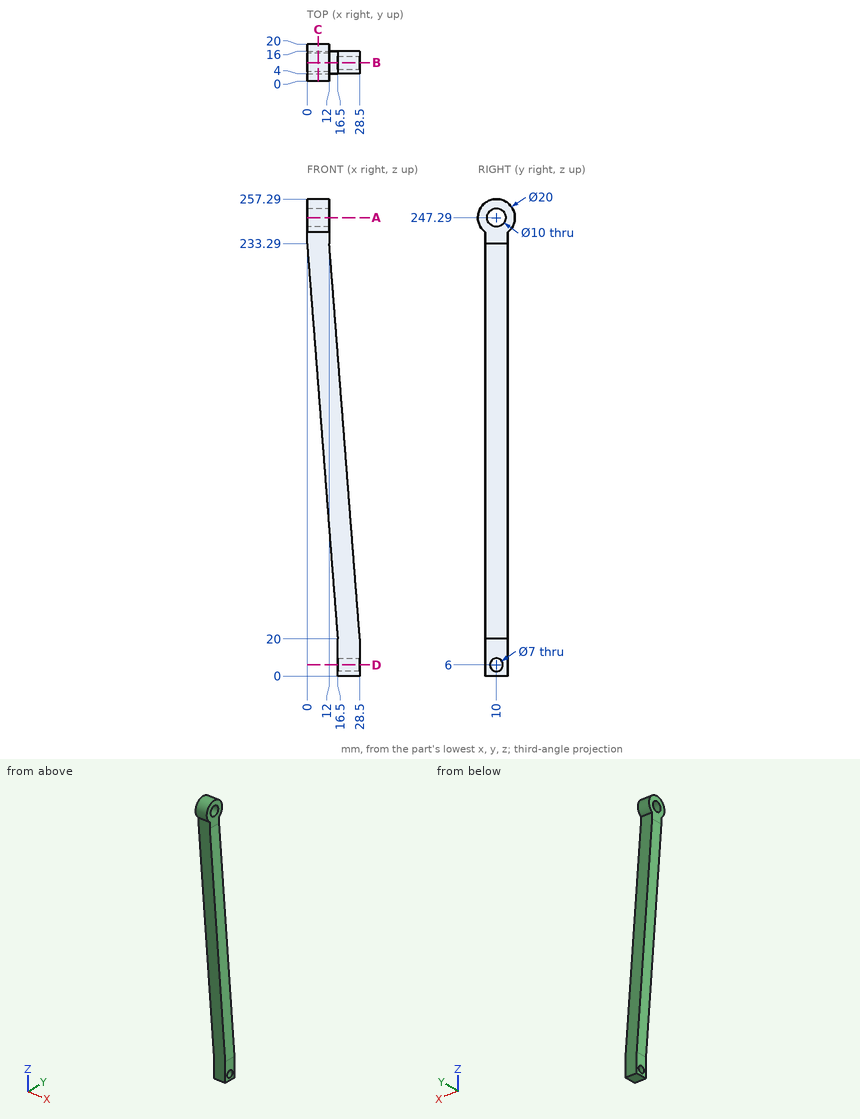
Answer from the drawing. Dimensions are ordinates in mm from the lowest x, y and z of the part. Round coordinates to 2 decimals unless told otherwise and drop trailing zeros. Write each loop counter-clockwise with the first axis right and the second up, starting at its lowest first coordinate (ties: lowest second). Pieces come first, ordered by that corner, then holes.
1. The part is cut by section C-C, the plane x = 6. Determine the outline of the cut face in (y, z).
2. Straight lines are drawn through the part: L1, parallel to Y at x = 25.5, z = 6; L2, parallel to Y at x = 4.5, z = 247.29; L3, parallel to Y at x = 9, z = 141. For each, find the intervals that lie inside material, in ascending order.
3. The part is cut by section D-D, the plane z = 6. Determine the outline of the cut face in (x, y).
4. The part is cut by section A-A, the plane z = 247.29. Determine the outline of the cut face in (x, y), then the cut area to 3 significant figures.
5. The part is cut by section B-B, the plane y = 10. Determine the outline of the cut face in (x, z), then the cut area to 3 significant figures.
6. Given pin 1 Ø3 at (x, z) = (12.5, 163) entering from +Y; pin 2 Ø9.5 at (y, z) = (8, 13.5) entering from -X; pin 3 Ø10 at (y, z) = (10, 246.5) entering from +X, each flat-ended and moving along its own axis, determine where each tip first touches the part or whether it passes through.
Values:
1. outline: (4, 155.73) - (16, 155.73) - (16, 239.29) arc R10 ccw (long way) to (4, 239.29) - close; hole circle Ø10 at (10, 247.29)
2. L1: y = 4 to 6.5, 13.5 to 16
2. L2: y = 0 to 5, 15 to 20
2. L3: y = 4 to 16
3. outline: (16.5, 4) - (28.5, 4) - (28.5, 6.5) - (16.5, 6.5) - close; (16.5, 13.5) - (28.5, 13.5) - (28.5, 16) - (16.5, 16) - close
4. outline: (0, 0) - (12, 0) - (12, 5) - (0, 5) - close; (0, 15) - (12, 15) - (12, 20) - (0, 20) - close
4. area: 120 mm2
5. outline: (0, 233.29) - (16.5, 20) - (16.5, 9.5) - (28.5, 9.5) - (28.5, 20) - (12, 233.29) - (12, 242.29) - (0, 242.29) - close; (0, 252.29) - (12, 252.29) - (12, 257.29) - (0, 257.29) - close; (16.5, 0) - (28.5, 0) - (28.5, 2.5) - (16.5, 2.5) - close
5. area: 2,880 mm2
6. pin 1: stops at y = 16
6. pin 2: stops at x = 16.5
6. pin 3: stops at x = 12
